Input: part model. Units: mm. Frame: model coordinates. Round coordinates to 2 decimals unless told otherwise and drop trailing zeros. Write each loop counter-clockwise with the first axis right and the second up, starting at its lowest first coordinate (ties: lowest second). Pieces come first, ordered by that corner, then holes. Notation, with made-up numbers: M 5.25,45.25 L 62.25,45.25 A25 cw 62.25,71.25 Z; hole C -28,2.5 d2. An arc over 180 degrees is marked long. Answer as CSV lines item,"result". Start each with the question number.
```python
from build123d import *

# Parameters (mm, degrees)
F0_R     = 12.7
F0_R_2   = 5.08
F1_DEPTH = 76.2
F2_DEPTH = 76.2
F3_SIZE  = 5.08


with BuildPart() as f1:
    # F0 (on Front) → F1 (new body)
    with BuildSketch(Plane.XZ):
        Circle(F0_R)
        Circle(F0_R_2, mode=Mode.SUBTRACT)
    extrude(amount=F1_DEPTH)

    # F0 (on Front) → F2 (join)
    with BuildSketch(Plane.XZ):
        Circle(F0_R_2)
    extrude(amount=F2_DEPTH)

    # F3
    f3_edges = [f1.edges().sort_by_distance(p)[0] for p in [
        (-12.7, -76.2, 0),
        (-12.7, 0, 0),
    ]]
    chamfer(f3_edges, length=F3_SIZE)


solid = f1.part
```
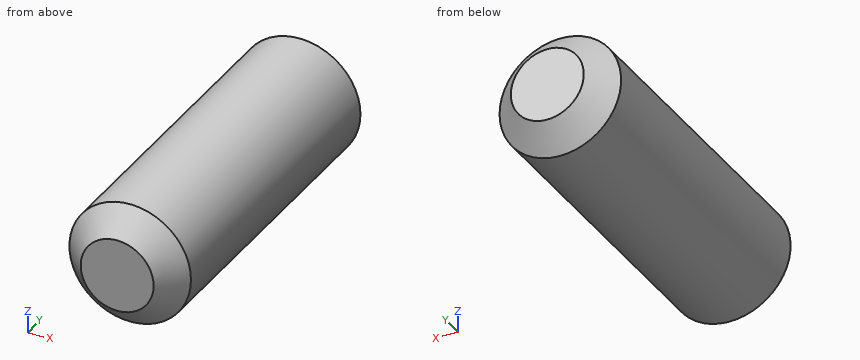
Item 1: Cut plane A-A, the plane z = 0. Return loops of the section in (x, y).
Item 2: Line query: line 1 (X direction, y = -18.5, z = -0.5); line 2 (Y direction, x = 9.5, z = -8); line 3 (Z direction, x = -7.25, y = -47). Output: solid intervals per line, ascending. Write a range as [from, to].
Item 3: Cut plane C-C, the plane y = -65.5. Return loops of the section in (x, z).
Item 4: Cut plane B-B, the plane x = 0. Return loops of the section in (y, z).
Item 5: Pin query (flat end, axial travel): pin 1 Ø5 at (x, y) = (7.5, -40.5) entering from +Z; pin 2 Ø2 at (x, y) = (-6.5, -46) entering from +Z; pin 3 Ø10 at (y, z) = (-44, -6.5) entering from +X. Return the tip coordinate at first contact, or that it passes through.
Results list:
1,outline,"M -12.7,-71.12 L -7.62,-76.2 L 7.62,-76.2 L 12.7,-71.12 L 12.7,-5.08 L 7.62,0 L -7.62,0 L -12.7,-5.08 Z"
2,line 1,"[-12.69, 12.69]"
2,line 2,"[-71.4, -4.8]"
2,line 3,"[-10.43, 10.43]"
3,outline,"C 0,0 d25.4"
4,outline,"M -76.2,-7.62 L -71.12,-12.7 L -5.08,-12.7 L 0,-7.62 L 0,7.62 L -5.08,12.7 L -71.12,12.7 L -76.2,7.62 Z"
5,pin 1,"z = 11.67"
5,pin 2,"z = 11.45"
5,pin 3,"x = 12.61"
